The listing builds one solid part. Answer for the finished solid, in the listing's coordinates (mm). A direction names the side the tool comes from. Round coordinates to 2 decimals unless told otherwise and drop trailing zeros. Write each loop counter-clockwise with the first axis right and the second up, starting at its lowest first coordinate (ties: lowest second). Pieces come first, ordered by that corner, then holes.
(1) A cutting plane is placed at B-B, the plane z = 4. Give the vertices of the cut face in (x, y), and give its area (3 significant figures).
(2) Find the intervals of material crossed by probe 1 along Z at (x, y) = (6, -27.3); probe 2 along Y at (x, z) = (3.75, 19); probe 3 along Y at (x, z) = (-0.25, 9), in increasing order.
(3) A cutting plane is placed at A-A, the plane x = -4. Give the vertices of the cut face in (y, z).
(4) Each of these flat-tipped pins is pushed along its axis until it touches: pin 1 Ø12 at (y, z) = (-6.5, 11) entering from -X; pin 2 Ø16.5 at (y, z) = (-12.5, 7) entering from +X; pin 3 Ø3.5 at (x, y) = (3, 17) entering from +Z. Where does it stop, or does it pass through?
(5) A cutting plane is placed at D-D, the plane x = 2.25. Give the vertices of the cut face in (y, z).
(6) The mould has two halves that part along Z. Classify faces 1 (the face through (4, 18, 15)), 2 (the face through (6, -8, 2)), 3 (the face through (-4, -11, 10)): +Z half, -Z half, draft (parallel to the pull), parting line (faces both ways), or undercut.
(7) For faces 4 (the face through (0, -16, 15)), 5 (the face through (1.5, 19, 9)), 6 (the face through (4, -8, 9)), 7 (the face through (-6, -8, 2)), determine the directions among +Z, -Z, +X, -X, +Y, -Y from which every point of the face is accessible in a straight line to the end or side of a thin tool.
(8) A cutting plane is placed at C-C, the plane y = -10.25. Give the vertices of the cut face in (x, z).
from build123d import *

# Parameters (mm, degrees)
SKETCH_1_W          = 12
SKETCH_1_H          = 40
EXTRUDE_1_DEPTH     = 3
SKETCH_2_W          = 4.5
SKETCH_2_H          = 5
SKETCH_2_W_2        = 4.7
EXTRUDE_2_DEPTH     = 12
SKETCH_3_R          = 1.25
CUT_EXTRUDE_1_DEPTH = 12
SKETCH_4_W          = 12
SKETCH_4_H          = 15
EXTRUDE_3_DEPTH     = 8
SKETCH_5_W          = 12
SKETCH_5_H          = 3
EXTRUDE_4_DEPTH     = 25
SKETCH_6_W          = 40
SKETCH_6_H          = 3
EXTRUDE_5_DEPTH     = 3
SKETCH_7_R          = 1.65
CUT_EXTRUDE_2_DEPTH = 3
SKETCH_8_W          = 40
SKETCH_8_H          = 3
EXTRUDE_6_DEPTH     = 3


with BuildPart() as part:
    # 草图1 → 凸台-拉伸1 (new body)
    with BuildSketch(Plane.XY):
        Rectangle(SKETCH_1_W, SKETCH_1_H)
    extrude(amount=EXTRUDE_1_DEPTH)

    # 草图2 → 凸台-拉伸2 (add)
    with BuildSketch(Plane.XY.offset(3)):
        with Locations((3.75, 17.5)):
            Rectangle(SKETCH_2_W, SKETCH_2_H)
        with Locations((-3.65, 17.5)):
            Rectangle(SKETCH_2_W_2, SKETCH_2_H)
        Polygon((-6, -8), (-1.3, -8), (-1.3, -13), (1.5, -13), (1.5, -8), (6, -8), (6, -20), (-6, -20), align=None)
    extrude(amount=EXTRUDE_2_DEPTH)

    # 草图3 → 切除-拉伸1 (cut)
    with BuildSketch(Plane(origin=(6, 0, 0), x_dir=(0, 0, -1), z_dir=(1, 0, 0))):
        with Locations(Location((-9, 17.25, 0), (0, 0, 90))):
            Circle(SKETCH_3_R)
        with Locations(Location((-9, -10.25, 0), (0, 0, 90))):
            Circle(SKETCH_3_R)
    extrude(amount=-CUT_EXTRUDE_1_DEPTH, mode=Mode.SUBTRACT)

    # 草图4 → 凸台-拉伸3 (add)
    with BuildSketch(Plane.XZ.offset(20)):
        with Locations((0, 7.5)):
            Rectangle(SKETCH_4_W, SKETCH_4_H)
    extrude(amount=EXTRUDE_3_DEPTH)

    # 草图5 → 凸台-拉伸4 (add)
    with BuildSketch(Plane.XY.offset(15)):
        with Locations((0, -26.5)):
            Rectangle(SKETCH_5_W, SKETCH_5_H)
    extrude(amount=EXTRUDE_4_DEPTH)

    # 草图6 → 凸台-拉伸5 (add)
    with BuildSketch(Plane(origin=(6, 0, 0), x_dir=(0, 0, -1), z_dir=(1, 0, 0))):
        with Locations((-20, -26.5)):
            Rectangle(SKETCH_6_W, SKETCH_6_H)
    extrude(amount=EXTRUDE_5_DEPTH)

    # 草图7 → 切除-拉伸2 (cut)
    with BuildSketch(Plane(origin=(0, -25, 0), x_dir=(1, 0, 0), z_dir=(0, 1, 0))):
        with Locations(Location((6, -23, 0), (0, 0, 180))):
            Circle(SKETCH_7_R)
        with Locations(Location((6, -33, 0), (0, 0, 180))):
            Circle(SKETCH_7_R)
        with Locations(Location((-4, -23, 0), (0, 0, 180))):
            Circle(SKETCH_7_R)
        with Locations(Location((-4, -33, 0), (0, 0, 180))):
            Circle(SKETCH_7_R)
    extrude(amount=-CUT_EXTRUDE_2_DEPTH, mode=Mode.SUBTRACT)

    # 草图8 → 凸台-拉伸6 (add)
    with BuildSketch(Plane.ZY.offset(6)):
        with Locations((20, -26.5)):
            Rectangle(SKETCH_8_W, SKETCH_8_H)
    extrude(amount=EXTRUDE_6_DEPTH)


solid = part.part
Solutions:
1. outline: (-9, -28) - (9, -28) - (9, -25) - (6, -25) - (6, -8) - (1.5, -8) - (1.5, -13) - (-1.3, -13) - (-1.3, -8) - (-6, -8) - (-6, -25) - (-9, -25) - close; (-6, 15) - (-1.3, 15) - (-1.3, 20) - (-6, 20) - close; (1.5, 15) - (6, 15) - (6, 20) - (1.5, 20) - close
1. area: 290 mm2
2. probe 1: z = 0 to 21.35, 24.65 to 31.35, 34.65 to 40
2. probe 2: y = -28 to -25
2. probe 3: y = -28 to -13
3. outline: (-28, 0) - (20, 0) - (20, 15) - (15, 15) - (15, 3) - (-8, 3) - (-8, 15) - (-25, 15) - (-25, 21.35) - (-28, 21.35) - close; (-28, 24.65) - (-25, 24.65) - (-25, 31.35) - (-28, 31.35) - close; (-28, 34.65) - (-25, 34.65) - (-25, 40) - (-28, 40) - close; hole circle Ø2.5 at (-10.25, 9); hole circle Ø2.5 at (17.25, 9)
4. pin 1: stops at x = -6
4. pin 2: stops at x = 6
4. pin 3: stops at z = 15
5. outline: (-28, 0) - (20, 0) - (20, 15) - (15, 15) - (15, 3) - (-8, 3) - (-8, 15) - (-25, 15) - (-25, 40) - (-28, 40) - close; hole circle Ø2.5 at (-10.25, 9); hole circle Ø2.5 at (17.25, 9)
6. face 1: +Z half
6. face 2: draft
6. face 3: undercut
7. face 4: +Z, +X, -X, +Y
7. face 5: +Z, +Y
7. face 6: +Z, +X, -X
7. face 7: +Z, -Z, -X, +Y
8. outline: (-6, 0) - (6, 0) - (6, 7.75) - (1.5, 7.75) - (1.5, 3) - (-1.3, 3) - (-1.3, 7.75) - (-6, 7.75) - close; (-6, 10.25) - (-1.3, 10.25) - (-1.3, 15) - (-6, 15) - close; (1.5, 10.25) - (6, 10.25) - (6, 15) - (1.5, 15) - close
